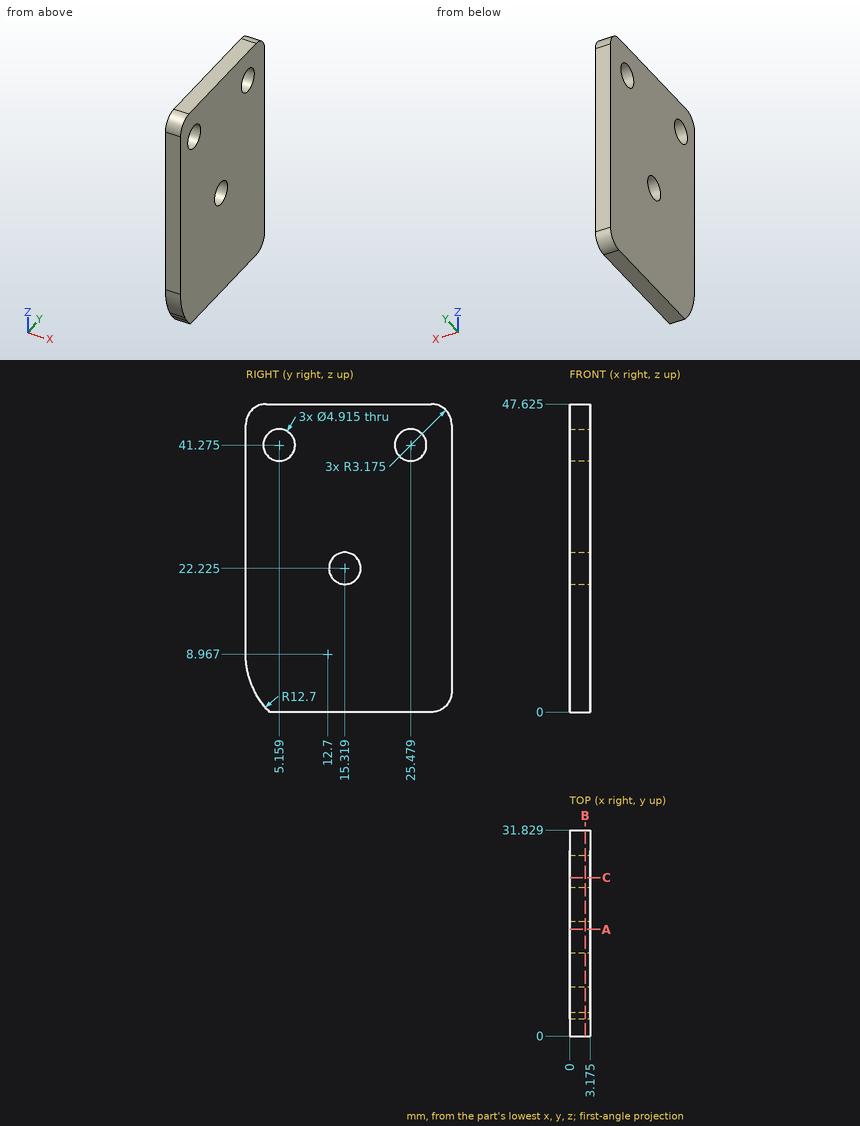
For this review, use the dimensioned drawing (mm, ordinates from the lowest corner) and the shaded views. Give positions to 0.01 mm unless a question says otherwise; leave off trailing zeros. Loops run counter-clockwise (first coordinate to the right, second up) from the corner with the lowest first, then second, coordinate; pieces in that order, holes last. Notation, with made-up numbers: (-25, -25) -> (-5, -25) arc R19 cw to (-5, -13) -> close; hole circle Ø10 at (84.25, 60). An arc over 180 degrees is marked (long way). One line per question, with ' | ' between items. Start each with the question number.
(1) We need section A-A (y = 16.5). State the section outline as (x, z) points (1 decimal).
(2) Insertion check: P1, Ø5.5, axis at y = 15.32, z = 22.23, coming from the +X side (3 decimals). The pin has a flat end and moves straight along its axis. Give the tip position at first contact, or say it passes through.
(3) We need section B-B (x = 2.4). State how many separate pieces and enclosed holes the cut face has, and give its area (3 significant figures).
(4) We need section C-C (y = 24.5). State the section outline as (x, z) points (3 decimals), and give its area (3 significant figures).
(5) For line 1 (Y direction, x = 0.75, z = 42); line 2 (Z direction, x = 2, y = 5.5) (1 decimal); line 3 (Y direction, x = 1.4, z = 20) (1 decimal), list the stretches that pass through material, from the lowest coordinate up.
The answers:
1) outline: (0, 0) -> (3.2, 0) -> (3.2, 20.1) -> (0, 20.1) -> close; (0, 24.4) -> (3.2, 24.4) -> (3.2, 47.6) -> (0, 47.6) -> close
2) P1: stops at x = 3.175
3) separate pieces: 1 | enclosed holes: 3 | area: 1,440 mm^2
4) outline: (0, 0) -> (3.175, 0) -> (3.175, 39.021) -> (0, 39.021) -> close; (0, 43.529) -> (3.175, 43.529) -> (3.175, 47.625) -> (0, 47.625) -> close | area: 137 mm^2
5) line 1: y = 0 to 2.81, 7.51 to 23.13, 27.83 to 31.83 | line 2: z = 0 to 38.8, 43.7 to 47.6 | line 3: y = 0 to 14.3, 16.4 to 31.8
